The listing builds one solid part. Answer for the finished solid, in the listing's coordinates (mm). A direction names the side the tool comes from. Give positions to 0.01 mm unless a question says otherwise; leave off trailing zeros. Order: outer loops, then holes, each group sorted by start corner. A loop starts at its lowest first (then second) coordinate and runs counter-clockwise, first axis right, second up. Notation, with made-up numbers: (-28, 80.5) - (-4, 80.5) arc R18 cw to (-4, 93.5) - close; hole circle Ø3 at (61, 82.5). An arc over 180 degrees is marked (long way). Answer as a JSON object with one key per item and string values. Group by question number.
Q1. Given pin 1 (10.5 mm diameter, centred on x = 30, y = 30, fed in from -Z); pin 2 (9.5 mm diameter, centred on x = -19.05, y = 11, fed in from +Z), each flat-ended and moving along its own axis, determine where each tip first touches the part or whether it passes through.
Q2. A cutting plane is placed at A-A, the plane z = 5.75. Count the separate pieces of the cut face and the enclosed holes in it, and give its area (3 significant figures).
Q3. A cutting plane is placed at D-D, the plane x = -15.5. Give the vertices of the cut face in (y, z), and give its area (3 significant figures).
Q4. The mould has two halves that part along X. Classify faces 1 (the face through (5.589, -2.317, 5.535)), 2 (the face through (-23, -27.1, 0.5)): released by +X, released by -X, zero draft, split by the parting line, or undercut.
Q5. Consider line 1 (Y direction, x = -30, z = 0.5) (3 decimals); line 2 (Y direction, x = 0, z = 2.35). Determine where each line is inside the solid, lowest interval first.
Q6. For faces 3 (the face through (-1.19, -5.37, 1.52)), 4 (the face through (-27, 33, 1)), 5 (the face through (-20.35, 5.14, 5.54)), determine the directions among +Z, -Z, +X, -X, +Y, -Y from which every point of the face is accessible in a straight line to the end or side of a thin tool.
Q7. A cutting plane is placed at B-B, the plane y = -30. Give the vertices of the cut face in (x, z) (3 decimals), and give its area (3 significant figures).
Q8. A cutting plane is placed at C-C, the plane x = 0. Give the vertices of the cut face in (y, z), and give its area (3 significant figures).
from build123d import *

# Parameters (mm, degrees)
F0_W     = 80
F0_H     = 80
F1_DEPTH = 8
F2_R     = 5.5
F2_R_2   = 4
F3_DEPTH = 25
F4_R     = 6
F4_R_2   = 6.05
F5_DEPTH = 5
F6_R     = 7.575
F7_DEPTH = 1


with BuildPart() as f1:
    # F0 (on Top) → F1 (new body)
    with BuildSketch(Plane.XY):
        Rectangle(F0_W, F0_H)
    extrude(amount=F1_DEPTH)

    # F2 (on face) → F3 (cut)
    with BuildSketch(Plane.XY.offset(8)):
        with Locations((-19.052559, 11)):
            Circle(F2_R)
        with Locations((-30, 30)):
            Circle(F2_R_2)
        with Locations((19.052559, 11)):
            Circle(F2_R)
        with Locations((30, 30)):
            Circle(F2_R_2)
        with Locations((30, -30)):
            Circle(F2_R_2)
        with Locations((0, -22)):
            Circle(F2_R)
        with Locations((-30, -30)):
            Circle(F2_R_2)
        Circle(F2_R)
    extrude(amount=-F3_DEPTH, mode=Mode.SUBTRACT)

    # F4 (on face) → F5 (cut)
    with BuildSketch(Plane.XY.offset(8)):
        with Locations((-19.052559, 11)):
            Circle(F4_R)
        with Locations((19.052559, 11)):
            Circle(F4_R_2)
        Circle(F4_R_2)
        with Locations((0, -22)):
            Circle(F4_R_2)
    extrude(amount=-F5_DEPTH, mode=Mode.SUBTRACT)

    # F6 (on face) → F7 (cut)
    with BuildSketch(Plane(origin=(0, 0, 0), x_dir=(1, 0, 0), z_dir=(0, 0, -1))):
        with Locations((-30, 30)):
            Circle(F6_R)
        with Locations((30, 30)):
            Circle(F6_R)
        with Locations((30, -30)):
            Circle(F6_R)
        with Locations((-30, -30)):
            Circle(F6_R)
    extrude(amount=-F7_DEPTH, mode=Mode.SUBTRACT)


solid = f1.part
Reply:
{
 "1": {"pin 1": "stops at z = 1", "pin 2": "passes through"},
 "2": {"separate pieces": "1", "enclosed holes": "8", "area": "5,740 mm^2"},
 "3": {"outline": "(-40, 0) - (6.8, 0) - (6.8, 3) - (6.16, 3) - (6.16, 8) - (-40, 8) - close; (15.2, 0) - (40, 0) - (40, 8) - (15.84, 8) - (15.84, 3) - (15.2, 3) - close", "area": "566 mm^2"},
 "4": {"face 1": "undercut", "face 2": "undercut"},
 "5": {"line 1": "y = -40 to -37.575, -22.425 to 22.425, 37.575 to 40", "line 2": "y = -40 to -27.5, -16.5 to -5.5, 5.5 to 40"},
 "6": {"face 3": "+Z, -Z", "face 4": "-Z", "face 5": "+Z"},
 "7": {"outline": "(-40, 0) - (-37.575, 0) - (-37.575, 1) - (-34, 1) - (-34, 8) - (-40, 8) - close; (-26, 1) - (-22.425, 1) - (-22.425, 0) - (22.425, 0) - (22.425, 1) - (26, 1) - (26, 8) - (-26, 8) - close; (34, 1) - (37.575, 1) - (37.575, 0) - (40, 0) - (40, 8) - (34, 8) - close", "area": "498 mm^2"},
 "8": {"outline": "(-40, 0) - (-27.5, 0) - (-27.5, 3) - (-28.05, 3) - (-28.05, 8) - (-40, 8) - close; (-16.5, 0) - (-5.5, 0) - (-5.5, 3) - (-6.05, 3) - (-6.05, 8) - (-15.95, 8) - (-15.95, 3) - (-16.5, 3) - close; (5.5, 0) - (40, 0) - (40, 8) - (6.05, 8) - (6.05, 3) - (5.5, 3) - close", "area": "453 mm^2"}
}
